For this review, take the finished solid that the model builds, in its own axes (mm). Face numbers are marked on the shaded views. A direction names the side the tool comes from. Coordinates: 2 decimals unless noted, no trailing zeros. Write each loop counter-clockwise with the first axis right and the second up, starting at its lowest first coordinate (ties: lowest second). Pieces come first, ordered by that corner, then holes.
```python
from build123d import *

# Parameters (mm, degrees)
SKETCH2_R           = 0.85
BOSS_EXTRUDE1_DEPTH = 4
SKETCH3_W           = 16.2
SKETCH3_H           = 19.455
CUT_EXTRUDE1_DEPTH  = 2


with BuildPart() as part:
    # Sketch2 → Boss-Extrude1 (new body)
    with BuildSketch(Plane.XY):
        with BuildLine():
            Line((0, 7), (0, 12.455))
            Line((0, 12.455), (4, 12.455))
            Line((4, 12.455), (4, 14.455))
            Line((4, 14.455), (0, 14.455))
            Line((0, 14.455), (0, 17.455))
            ThreePointArc((0, 17.455), (0.585786438, 18.869213562), (2, 19.455))
            Line((2, 19.455), (14.2, 19.455))
            ThreePointArc((14.2, 19.455), (15.614213562, 18.869213562), (16.2, 17.455))
            Line((16.2, 17.455), (16.2, 14.455))
            Line((16.2, 14.455), (12.2, 14.455))
            Line((12.2, 14.455), (12.2, 12.455))
            Line((12.2, 12.455), (16.2, 12.455))
            Line((16.2, 12.455), (16.2, 7))
            Line((16.2, 7), (12.2, 7))
            Line((12.2, 7), (12.2, 5))
            Line((12.2, 5), (16.2, 5))
            Line((16.2, 5), (16.2, 2))
            ThreePointArc((16.2, 2), (15.614213562, 0.585786438), (14.2, 0))
            Line((14.2, 0), (2, 0))
            ThreePointArc((2, 0), (0.585786438, 0.585786438), (0, 2))
            Line((0, 2), (0, 5))
            Line((0, 5), (4, 5))
            Line((4, 5), (4, 7))
            Line((4, 7), (0, 7))
        make_face()
        with Locations((13.45, 2.5)):
            Circle(SKETCH2_R, mode=Mode.SUBTRACT)
        with Locations((2.75, 16.955)):
            Circle(SKETCH2_R, mode=Mode.SUBTRACT)
        with Locations((2.75, 2.5)):
            Circle(SKETCH2_R, mode=Mode.SUBTRACT)
        with Locations((13.45, 16.955)):
            Circle(SKETCH2_R, mode=Mode.SUBTRACT)
    extrude(amount=BOSS_EXTRUDE1_DEPTH)

    # Sketch3 → Cut-Extrude1 (cut)
    with BuildSketch(Plane.XY.offset(4)):
        with Locations((8.1, 9.7275)):
            Rectangle(SKETCH3_W, SKETCH3_H)
    extrude(amount=-CUT_EXTRUDE1_DEPTH, mode=Mode.SUBTRACT)


solid = part.part
```
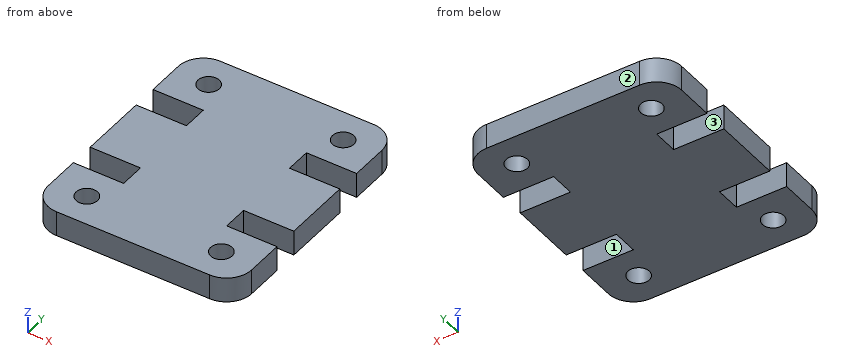
Q1. Clearance check with flat-ended pins moving along their axes: pin 1 Ø1 at (x, z) = (13.5, 1) entering from -Y; pin 2 Ø1 at (x, y) = (2.75, 16.955) entering from +Z; pin 3 Ø1 at (x, z) = (15, 1) entering from +Y. State where each tip first meets the part, or that it passes through.
Ans:
pin 1: stops at y = 0
pin 2: passes through
pin 3: stops at y = 19.43
Q2. For probe 1 along Y at (x, z) = (2.75, 1.15) (3 decimals); probe 2 along X at (y, z) = (2.5, 1.3); probe 3 along X at (y, z) = (1.75, 0.6), list the stretches that pass through material, from the lowest coordinate up.
Ans:
probe 1: y = 0 to 1.65, 3.35 to 5, 7 to 12.455, 14.455 to 16.105, 17.805 to 19.455
probe 2: x = 0 to 1.9, 3.6 to 12.6, 14.3 to 16.2
probe 3: x = 0.02 to 2.35, 3.15 to 13.05, 13.85 to 16.18
Q3. Add section B-B (x = 2.75). State the section outline as (y, z) points (3 decimals), then the cut area to 3 significant figures.
Ans:
outline: (0, 0) - (1.65, 0) - (1.65, 2) - (0, 2) - close; (3.35, 0) - (5, 0) - (5, 2) - (3.35, 2) - close; (7, 0) - (12.455, 0) - (12.455, 2) - (7, 2) - close; (14.455, 0) - (16.105, 0) - (16.105, 2) - (14.455, 2) - close; (17.805, 0) - (19.455, 0) - (19.455, 2) - (17.805, 2) - close
area: 24.1 mm2
Q4. Add section A-A (y = 2.5). State the section outline as (x, z) points, then the cut area to 3 significant figures.
Ans:
outline: (0, 0) - (1.9, 0) - (1.9, 2) - (0, 2) - close; (3.6, 0) - (12.6, 0) - (12.6, 2) - (3.6, 2) - close; (14.3, 0) - (16.2, 0) - (16.2, 2) - (14.3, 2) - close
area: 25.6 mm2
Q5. Tool access review of the marked faces 1, 2 and 3: name each direction out of +Z, -Z, +X, -X, +Y, -Y from which nothing blocks a thin tool from reaching the whole face with its end or side.
Ans:
face 1: +Z, -Z, +X
face 2: +Z, -Z, +X, -X, +Y
face 3: +Z, -Z, -X
Q6. Add section C-C (z = 0.8). State the section outline as (x, y) points (3 decimals), then the cut area to 3 significant figures.
Ans:
outline: (0, 2) arc R2 ccw to (2, 0) - (14.2, 0) arc R2 ccw to (16.2, 2) - (16.2, 5) - (12.2, 5) - (12.2, 7) - (16.2, 7) - (16.2, 12.455) - (12.2, 12.455) - (12.2, 14.455) - (16.2, 14.455) - (16.2, 17.455) arc R2 ccw to (14.2, 19.455) - (2, 19.455) arc R2 ccw to (0, 17.455) - (0, 14.455) - (4, 14.455) - (4, 12.455) - (0, 12.455) - (0, 7) - (4, 7) - (4, 5) - (0, 5) - close; hole circle Ø1.7 at (2.75, 2.5); hole circle Ø1.7 at (2.75, 16.955); hole circle Ø1.7 at (13.45, 2.5); hole circle Ø1.7 at (13.45, 16.955)
area: 271 mm2
Q7. Add section D-D (x = 13.75). State the section outline as (y, z) points (3 decimals).
Ans:
outline: (0, 0) - (1.705, 0) - (1.705, 2) - (0, 2) - close; (3.295, 0) - (5, 0) - (5, 2) - (3.295, 2) - close; (7, 0) - (12.455, 0) - (12.455, 2) - (7, 2) - close; (14.455, 0) - (16.16, 0) - (16.16, 2) - (14.455, 2) - close; (17.75, 0) - (19.455, 0) - (19.455, 2) - (17.75, 2) - close
